The listing builds one solid part. Answer for the finished solid, in the listing's coordinates (mm). A direction names the side the tool comes from. Coordinates: 2 decimals unless noted, no trailing zeros. Order: outer loops, then holes, each group sorted by start corner. A loop starts at its lowest first (then second) coordinate and runs counter-clockwise, first axis right, second up. Notation, with made-up numbers: (-14, -31) -> (45, -31) arc R12 ccw to (45, -13) -> close; hole circle Ø4 at (-16, 8.25). An arc over 180 degrees is marked (long way). Answer in a Markdown table with one row per item.
```python
from build123d import *

# Parameters (mm, degrees)
F0_W           = 479.75
F0_H           = 130
F1_DEPTH       = 14
F2_W           = 20
F2_H           = 10
F3_DEPTH       = 130
F4_W           = 11
F4_H           = 16
F5_DEPTH       = 130
F6_W           = 42.5000000004
F6_H           = 18.3330895797
F6_W_2         = 42.5
F6_H_2         = 67.2669104207
F6_H_3         = 18.3330895795
F6_W_3         = 42.4708837634
F6_H_4         = 67.2961863439
F6_W_4         = 42.5291162366
F6_H_5         = 67.2961863442
F6_W_5         = 42.4708837635
F7_DEPTH       = 25
F8_R           = 2.5
F9_DEPTH       = 25
F10_R          = 2.5
F11_DEPTH      = 11.001
F11_DEPTH_BACK = 25
F12_R          = 2.5
F13_DEPTH      = 25
F14_SIZE       = 3.49999
F15_W          = 45
F15_H          = 20
F15_W_2        = 55
F15_H_2        = 15
F15_H_3        = 45
F16_DEPTH      = 25


# Not quite as in the source:
# - a fillet or chamfer is up to 0.001 mm smaller than in the source, because OpenCascade refuses the exact size
# - a feature names something its author has since deleted; it is built from what else it names


with BuildPart() as f1:
    # F0 (on Front) → F1 (new body)
    with BuildSketch(Plane.XZ):
        with Locations((239.875, 65)):
            Rectangle(F0_W, F0_H)
    extrude(amount=F1_DEPTH)

    # F2 (on face) → F3 (join, through all)
    with BuildSketch(Plane.XY.offset(130)):
        Polygon((479.75, 0), (479.75, -14), (509.75, -14), (509.75, 66), (479.75, 66), (479.75, 55), (495.75, 55), (495.75, 0), align=None)
        with Locations((-10, -9)):
            Rectangle(F2_W, F2_H)
    extrude(amount=-F3_DEPTH)

    # F4 (on face) → F5 (join, through all)
    with BuildSketch(Plane.XY.offset(130)):
        with Locations((5.5, 8)):
            Rectangle(F4_W, F4_H)
    extrude(amount=-F5_DEPTH)

    # F6 (on face) → F7 (cut)
    with BuildSketch(Plane.XZ.offset(14)):
        Polygon((21, 120), (21, 95), (11, 95), (11, 52.7330895796), (21, 52.7330895796), (63.5, 52.7330895796), (63.5, 120), align=None)
        with Locations((42.2499999998, 19.1665447897)):
            Rectangle(F6_W, F6_H)
        with Locations((109.15, 43.6334552101)):
            Rectangle(F6_W_2, F6_H_2)
        with Locations((151.65, 43.6334552101)):
            Rectangle(F6_W_2, F6_H_2)
        with Locations((109.15, 110.8334552102)):
            Rectangle(F6_W_2, F6_H_3)
        with Locations((151.65, 110.8334552102)):
            Rectangle(F6_W_2, F6_H_3)
        with Locations((218.5645581183, 86.351906828)):
            Rectangle(F6_W_3, F6_H_4)
        with Locations((261.0645581183, 86.351906828)):
            Rectangle(F6_W_4, F6_H_4)
        with Locations((218.5645581183, 19.1665447897)):
            Rectangle(F6_W_3, F6_H)
        with Locations((261.0645581183, 19.1665447897)):
            Rectangle(F6_W_4, F6_H)
        with Locations((328.0854418817, 43.6480931718)):
            Rectangle(F6_W_4, F6_H_5)
        with Locations((370.5854418817, 43.6480931718)):
            Rectangle(F6_W_5, F6_H_5)
        with Locations((370.5854418817, 110.8334552102)):
            Rectangle(F6_W_3, F6_H_3)
        with Locations((328.0854418817, 110.8334552102)):
            Rectangle(F6_W_4, F6_H_3)
        Polygon((458.75, 120), (416.25, 120), (416.25, 52.7330895795), (469.75, 52.7330895795), (469.75, 95), (458.75, 95), align=None)
        with Locations((437.5, 19.1665447897)):
            Rectangle(F6_W_2, F6_H)
    extrude(amount=-F7_DEPTH, mode=Mode.SUBTRACT)

    # F8 (on face) → F9 (cut)
    with BuildSketch(Plane(origin=(0, -4, 0), x_dir=(-1, 0, 0), z_dir=(0, 1, 0))):
        with Locations((10, 115)):
            Circle(F8_R)
        with Locations((10, 15)):
            Circle(F8_R)
    extrude(amount=-F9_DEPTH, mode=Mode.SUBTRACT)

    # F10 (on face) → F11 (cut, two sides)
    with BuildSketch(Plane.XZ.offset(-55)) as f11_sk:
        with Locations((489.75, 15)):
            Circle(F10_R)
        with Locations((489.75, 115)):
            Circle(F10_R)
    extrude(amount=-F11_DEPTH, mode=Mode.SUBTRACT)
    extrude(f11_sk.sketch, amount=F11_DEPTH_BACK, mode=Mode.SUBTRACT)

    # F12 (on face) → F13 (cut)
    with BuildSketch(Plane(origin=(0, 0, 0), x_dir=(0, -1, 0), z_dir=(-1, 0, 0))):
        with Locations((-6, 15)):
            Circle(F12_R)
        with Locations((-6, 115)):
            Circle(F12_R)
    extrude(amount=-F13_DEPTH, mode=Mode.SUBTRACT)

    # F14 (size 3.5 in the source; OpenCascade refuses exactly that, so slightly less here)
    f14_edges = [f1.edges().sort_by_distance(p)[0] for p in [
        (487.25, 55, 15),
        (487.25, 55, 115),
        (-7.5, -14, 15),
        (-7.5, -14, 115),
        (11, 8.5, 15),
        (11, 8.5, 115),
    ]]
    chamfer(f14_edges, length=F14_SIZE)

    # F15 (on face) → F16 (cut)
    with BuildSketch(Plane.YZ.offset(509.75)):
        with Locations((27.5, 20)):
            Rectangle(F15_W, F15_H)
        with Locations((27.5, 112.5)):
            Rectangle(F15_W_2, F15_H_2)
        with Locations((27.5, 67.5)):
            Rectangle(F15_W, F15_H_3)
    extrude(amount=-F16_DEPTH, mode=Mode.SUBTRACT)


solid = f1.part
```
(1) A cutting plane is placed at B-B, the plane x = 360. Determine the outline of the cut face in (y, z).
Check values:
| item | result |
|---|---|
| outline | (-14, 0) -> (0, 0) -> (0, 10) -> (-14, 10) -> close; (-14, 77.3) -> (0, 77.3) -> (0, 101.67) -> (-14, 101.67) -> close; (-14, 120) -> (0, 120) -> (0, 130) -> (-14, 130) -> close |
(2) A cutting plane is placed at D-D, the plane z = 39. Determine the outline of the cut face in (x, y).
Check values:
| item | result |
|---|---|
| outline | (-20, -14) -> (87.9, -14) -> (87.9, 0) -> (11, 0) -> (11, 16) -> (0, 16) -> (0, -4) -> (-20, -4) -> close; (172.9, -14) -> (306.82, -14) -> (306.82, 0) -> (172.9, 0) -> close; (391.82, -14) -> (509.75, -14) -> (509.75, 66) -> (479.75, 66) -> (479.75, 55) -> (495.75, 55) -> (495.75, 0) -> (391.82, 0) -> close |
(3) Find the intervals of material crossed by line 1 along Z through (x, y) = (489.75, 64); line 2 along Z through (x, y) = (36, -2.5); line 3 along X through (y, z) = (-4.5, 99.5), in increasing order. Write a range as from..to.
Check values:
| item | result |
|---|---|
| line 1 | 0..12.5, 17.5..112.5, 117.5..130 |
| line 2 | 0..10, 28.33..52.73, 120..130 |
| line 3 | -20..21, 63.5..197.33, 282.33..416.25, 458.75..509.75 |
(4) For a pull along X with two mould halves and no side action, classify faces 1 (the flat face through (263, -3, 130)), 2 (the flat face through (0, 6, 66)), 3 (the flat face through (197.329, -7, 19)) as released by +X, released by -X, zero draft, split by the parting line, or undercut.
Check values:
| item | result |
|---|---|
| face 1 | zero draft |
| face 2 | released by -X |
| face 3 | undercut |
(5) A cutting plane is placed at C-C, the plane y = 36.5. Determine the outline of the cut face in (x, z).
Check values:
| item | result |
|---|---|
| outline | (495.75, 0) -> (509.75, 0) -> (509.75, 10) -> (495.75, 10) -> close; (495.75, 30) -> (509.75, 30) -> (509.75, 45) -> (495.75, 45) -> close; (495.75, 90) -> (509.75, 90) -> (509.75, 105) -> (495.75, 105) -> close; (495.75, 120) -> (509.75, 120) -> (509.75, 130) -> (495.75, 130) -> close |
(6) A cutting plane is placed at A-A, the plane z = 70. Count the separate pieces of the cut face and the enclosed holes in it, then the cut area to 3 significant figures.
Check values:
| item | result |
|---|---|
| separate pieces | 7 |
| enclosed holes | 0 |
| area | 2,930 mm² |
(7) Flat-ended cylindrical pins translate along their axes: pin 1 (16 mm diameter, centred on y = 5, z = 35.5, fed in from -X); pin 2 (12 mm diameter, centred on x = 120.5, z = 112, fed in from +Y); pin 3 (6 mm diameter, centred on y = 26, z = 47, fed in from -X); pin 4 (3 mm diameter, centred on x = 489.75, z = 15, fed in from +Y). Find the tip coordinate at first contact, or state that the pin passes through.
Check values:
| item | result |
|---|---|
| pin 1 | x = 0 |
| pin 2 | through |
| pin 3 | x = 495.75 |
| pin 4 | y = 0 |
(8) Which of the six approach directions +Z, -Z, +X, -X, +Y, -Y give full straight-line access (tool end or side, diameter ignored) to faces 4 (the flat face through (503, 27, 10)), 5 (the flat face through (11, 4, 66)), 6 (the flat face through (349, -7, 101.667))?
Check values:
| item | result |
|---|---|
| face 4 | +X |
| face 5 | +Y |
| face 6 | +Y, -Y |
